Input: part model. Units: mm. Frame: model coordinates. Give positions to 0.01 mm unless a question says otherwise; leave off trailing zeros. Loops run counter-clockwise (first coordinate to the right, second up) from the corner with the lowest first, then second, coordinate; pieces in that order, holes last. Notation, with made-up numbers: (-27, -33) -> (32, -33) arc R7 cw to (32, -29) -> close; hole circle Ø3 at (-4, -16.5). An arc over 180 degrees is marked (long way). Use CSV: the item, a comma, the result in double quotes.
Autodesk Inventor part; units mm, degrees
ref_plane "YZ Plane" through (0, 0, 0) normal (1, 0, 0) x (0, 1, 0)
ref_plane "XZ Plane" through (0, 0, 0) normal (0, 1, 0) x (-1, 0, 0)
ref_plane "XY Plane" through (0, 0, 0) normal (0, 0, 1) x (1, 0, 0)
sketch "スケッチ1" plane through (0, 0, 0) normal (0, 0, 1) x (1, 0, 0)
  circle A0 centre (0, 0) radius 1.75
  circle A1 centre (0, 0) radius 3
  circle A2 centre (0, -53.1322) radius 1.75
  circle A3 centre (0, -53.1322) radius 3
  line L0 (0, 0) -> (0, -53.1322) construction
  circle A4 centre (0, -26.5661) radius 7.5
  line L1 (25, 29.4339) -> (-25, 29.4339)
  line L2 (-25, 29.4339) -> (-25, -82.5661)
  line L3 (-25, -82.5661) -> (25, -82.5661)
  line L4 (25, -82.5661) -> (25, 29.4339)
  line L5 (25, 29.4339) -> (-25, -82.5661) construction
  line L6 (-25, 29.4339) -> (25, -82.5661) construction
  line L7 (25, -26.5661) -> (0, -26.5661) construction
  circle A5 centre (-10, -79.6778) radius 0.7835
  point P0 (0, 0)
  point P1 (5, 29.4339)
  point P2 (-5, 29.4339)
  dimension "d0" = 6
  dimension "d1" = 6
  dimension "d2" = 15
  dimension "d4" = 50
  dimension "d14" = 112
extrude "押し出し1" add sketch "スケッチ1" along normal blind 1.5 contours L4 L3 L2 L1 | A5
sketch "スケッチ2" plane through (0, 0, 1.5) normal (0, 0, 1) x (1, 0, 0)
  line L0 (-5, -78.1778) -> (5, -78.1778)
  line L1 (-5, -81.1778) -> (5, -81.1778)
  line L2 (-5, -81.1778) -> (-5, -78.1778)
  line L3 (5, -81.1778) -> (5, -78.1778)
  circle A0 centre (-10, -79.6778) radius 0.7835
  circle A1 centre (10, -79.6778) radius 0.7835
  line L4 (5, 25.0456) -> (-5, 25.0456)
  line L5 (5, 28.0456) -> (-5, 28.0456)
  line L6 (-5, 28.0456) -> (-5, 25.0456)
  line L7 (5, 28.0456) -> (5, 25.0456)
  circle A2 centre (-10, 26.5456) radius 0.7835
  circle A3 centre (10, 26.5456) radius 0.7835
  circle A4 centre (3.9, -78.1778) radius 1.1
  line L8 (0, -78.1778) -> (0, -81.1778) construction
  line L9 (0, -79.6778) -> (-5, -79.6778) construction
  circle A5 centre (3.9, -81.1778) radius 1.1
  circle A6 centre (-3.9, -78.1778) radius 1.1
  circle A7 centre (-3.9, -81.1778) radius 1.1
  line L10 (-25, 29.4339) -> (-25, -82.5661) construction
  line L11 (-25, -26.5661) -> (25, -26.5661) construction
  line L12 (25, -82.5661) -> (25, 29.4339) construction
  circle A8 centre (3.9, 25.0456) radius 1.1
  circle A9 centre (3.9, 28.0456) radius 1.1
  circle A10 centre (-3.9, 28.0456) radius 1.1
  circle A11 centre (-3.9, 25.0456) radius 1.1
  circle A12 centre (-10, -79.6778) radius 1.1
  circle A13 centre (10, -79.6778) radius 1.1
  circle A14 centre (-10, 26.5456) radius 1.1
  circle A15 centre (10, 26.5456) radius 1.1
  point P0 (0, 0)
  point P1 (2.8, 25.0456)
  point P2 (-2.8, 25.0456)
  point P3 (-2.8, 28.0456)
  point P4 (2.8, -81.1778)
  point P5 (2.8, -78.1778)
  point P6 (-2.8, -81.1778)
  point P7 (-2.8, -78.1778)
  point P8 (2.8, 28.0456)
  dimension "d17" = 2.2
  dimension "d18" = 2.2
  dimension "d19" = 2.2
  dimension "d20" = 2.2
  dimension "d21" = 2.2
extrude "押し出し2" cut sketch "スケッチ2" against normal through all contours A6 L0 | A6 L0 A4 L3 A5 L1 A7 L2 | L0 A6 | A7 L1 | L1 A7 | A4 L0 | L0 A4 | A5 L1 | L1 A5 | A0 | A1 | A11 L4 | A11 L6 A10 L5 A9 L7 A8 L4 | L4 A11 | A8 L4 | L4 A8 | A10 L5 | L5 A10 | A9 L5 | L5 A9 | A2 | A3 | A12 | A13 | A14 | A15
properties part number "kosisita"
1) Section query C-C (x = -10). Return loops of the section in (y, z), then the cut area to 3 significant figures.
From the geometry:
outline,"(-82.57, 0) -> (-80.78, 0) -> (-80.78, 1.5) -> (-82.57, 1.5) -> close; (-78.58, 0) -> (25.45, 0) -> (25.45, 1.5) -> (-78.58, 1.5) -> close; (27.65, 0) -> (29.43, 0) -> (29.43, 1.5) -> (27.65, 1.5) -> close"
area,"161 mm^2"
2) Ray query, line 1 (Y direction, x = 10, z = 0.65); line 2 (Y direction, x = 0, z = 0.4); line 3 (X direction, y = -21, z = 1.35). Return the intervals inside material, ascending.
From the geometry:
line 1,"y = -82.57 to -80.78, -78.58 to 25.45, 27.65 to 29.43"
line 2,"y = -82.57 to -81.18, -78.18 to -56.13, -50.13 to -34.07, -19.07 to -3, 3 to 25.05, 28.05 to 29.43"
line 3,"x = -25 to -5.03, 5.03 to 25"
3) Mould query, pull axis Y, two halves, no side actions, for faces 1 (the flat face through (-11, -26, 1.5)), 2 (the cylindrical face through (10.508, -80.654, 0.76)). Classes: pulls with the +Y half, pulls with the -Y half, needs draft (parallel to the pull), parting line crosses it, or undercut.
From the geometry:
face 1,"needs draft"
face 2,"undercut"
4) Section query A-A (y = 0). Return loops of the section in (x, z), then the cut area to 3 significant figures.
From the geometry:
outline,"(-25, 0) -> (-3, 0) -> (-3, 1.5) -> (-25, 1.5) -> close; (3, 0) -> (25, 0) -> (25, 1.5) -> (3, 1.5) -> close"
area,"66.0 mm^2"
5) Section query B-B (x = 0.5). Return loops of the section in (y, z), then the cut area to 3 significant figures.
From the geometry:
outline,"(-82.57, 0) -> (-81.18, 0) -> (-81.18, 1.5) -> (-82.57, 1.5) -> close; (-78.18, 0) -> (-56.09, 0) -> (-56.09, 1.5) -> (-78.18, 1.5) -> close; (-50.17, 0) -> (-34.05, 0) -> (-34.05, 1.5) -> (-50.17, 1.5) -> close; (-19.08, 0) -> (-2.96, 0) -> (-2.96, 1.5) -> (-19.08, 1.5) -> close; (2.96, 0) -> (25.05, 0) -> (25.05, 1.5) -> (2.96, 1.5) -> close; (28.05, 0) -> (29.43, 0) -> (29.43, 1.5) -> (28.05, 1.5) -> close"
area,"119 mm^2"
6) Section query D-D (x = 6). Return loops of the section in (y, z), then the cut area to 4 significant figures.
From the geometry:
outline,"(-82.57, 0) -> (-31.07, 0) -> (-31.07, 1.5) -> (-82.57, 1.5) -> close; (-22.07, 0) -> (29.43, 0) -> (29.43, 1.5) -> (-22.07, 1.5) -> close"
area,"154.5 mm^2"
